Verification items for the finished model (mm, model axes). Face numbers are marked on the shaded views. A direction names the side the tool comes from. Round coordinates to 2 decimals unless told otherwise and drop trailing zeros. Write each loop counter-clockwise with the first axis right and the second up, starting at its lowest first coordinate (ties: lowest second). Pieces come first, ordered by that corner, then holes. Notation, with made-up numbers: M 15.5,34.25 L 20.5,34.25 A18 cw 20.5,59.25 Z; hole C 18.5,2 d11. An arc over 180 degrees is marked long. Write each question's results on one line, items separated by ' | '.
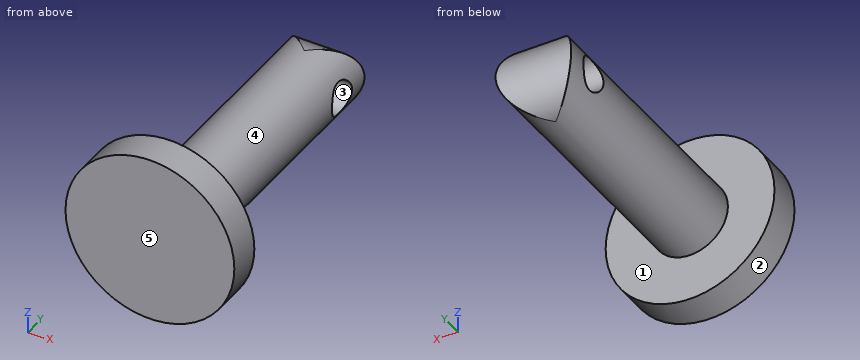
Autodesk Inventor part; units mm, degrees
ref_plane "YZ Plane" through (0, 0, 0) normal (1, 0, 0) x (0, 1, 0)
ref_plane "XZ Plane" through (0, 0, 0) normal (0, 1, 0) x (-1, 0, 0)
ref_plane "XY Plane" through (0, 0, 0) normal (0, 0, 1) x (1, 0, 0)
sketch "Sketch1" plane through (0, 0, 0) normal (0, 1, 0) x (-1, 0, 0)
  circle A0 centre (0, 0) radius 15.875
  circle A1 centre (0, 0) radius 7.112
  dimension "d0" = 31.75
  dimension "d1" = 14.224
extrude "Extrusion1" add sketch "Sketch1" along normal blind 50.8 contours A1
extrude "Extrusion2" add sketch "Sketch1" against normal blind 6.35 contours A0 | A1
sketch "Sketch2" plane through (0, 0, 0) normal (1, 0, 0) x (0, 1, 0)
  line L0 (50.8, -7.112) -> (50.8, 7.112)
  circle A0 centre (42.6249, 0) radius 3.175
  circle A1 centre (42.6249, 0) radius 7.112
  line L1 (0, -7.112) -> (50.8, -7.112)
  line L2 (42.6249, -7.112) -> (42.6249, -13.9262)
  line L3 (42.6249, -13.9262) -> (57.419, -13.9262)
  line L4 (57.419, -13.9262) -> (57.419, 14.0929)
  line L5 (57.419, 14.0929) -> (42.6249, 14.0929)
  line L6 (42.6249, 14.0929) -> (42.6249, 7.112)
  point P0 (0, 0)
  point P1 (39.4499, 0)
  dimension "d7" = 6.35
extrude "Extrusion3" cut sketch "Sketch2" along normal mid plane 127 contours A0 | A1 L6 L5 L4 L3 L2
properties part number "Load Cell Test Mount to Find Required Torque Application"
1) Sectioned sample at D-D, the plane x = 6. Record the cut outline in (y, z) (3 decimals).
Calculated:
outline: M -6.35,-14.697 L 0,-14.697 L 0,-3.818 L 48.625,-3.818 A7.112 ccw 48.625,3.818 L 0,3.818 L 0,14.697 L -6.35,14.697 Z; hole C 42.625,0 d6.35
2) Sectioned sample at B-B, the plane z = 0. Record the cut outline in (x, y) (3 decimals), and give its area (3 significant figures).
Calculated:
outline: M -15.875,-6.35 L 15.875,-6.35 L 15.875,0 L 7.112,0 L 7.112,39.45 L -7.112,39.45 L -7.112,0 L -15.875,0 Z; M -7.112,45.8 L 7.112,45.8 L 7.112,49.737 L -7.112,49.737 Z | area: 819 mm²
3) Sectioned sample at A-A, the plane x = 0. Record the cut outline in (y, z) (3 decimals).
Calculated:
outline: M -6.35,-15.875 L 0,-15.875 L 0,-7.112 L 42.625,-7.112 A7.112 ccw 42.625,7.112 L 0,7.112 L 0,15.875 L -6.35,15.875 Z; hole C 42.625,0 d6.35
4) Material ranges on line 1 (Y direction, x = -2, z = 0); line 2 (Z direction, x = 2.5, y = 41); line 3 (Y direction, x = -2, z = -12), recorded low to high. Write a range as [from, to].
Calculated:
line 1: y = [-6.35, 39.45], [45.8, 49.74] | line 2: z = [-6.66, -2.73], [2.73, 6.66] | line 3: y = [-6.35, 0]
5) Access from +Z, -Z, +X, -X, +Y, -Y to the whole of each face (thin tool, end or side, straight path). Record for the marked faces 4 and 5.
Calculated:
face 4: +Y | face 5: +Z, -Z, +X, -X, -Y
6) Sectioned sample at C-C, the plane y = 3.5. Record the cut outline in (x, z), and give its area (3 significant figures).
Calculated:
outline: C 0,0 d14.22 | area: 159 mm²
7) Depth check by flat-ended pin: P1, Ø12, axis at x = 7.5, z = -9, coming from the +Y side; P2, Ø8, axis at x = 7.5, y = 14, coming from the -Z side; P3, Ø2, axis at y = 26, z = -5, coming from the -X side. Enter the tip coordinate at first touch or a pass-through.
Calculated:
P1: stops at y = 49.02 | P2: stops at z = -6.19 | P3: stops at x = -5.88
8) Draft check along Z on the marked faces 1, 2 and 3. Enter one of: pulls with the +Z half, pulls with the -Z half, needs draft (parallel to the pull), parting line crosses it, or undercut.
Calculated:
face 1: needs draft | face 2: parting line crosses it | face 3: undercut
